Input: part model. Units: mm. Frame: model coordinates. Face numbers are marked on the shaded views. A direction names the side the tool comes from. Round coordinates to 2 decimals unless told otherwise and drop trailing zeros. Loops run counter-clockwise (first coordinate to the right, second up) from the corner with the lowest first, then second, coordinate; pieces in that order, holes last.
1) First-contact query: pin 1 (5 mm diameter, centred on y = -2, z = 13.5, fed in from -X); pin 2 (3 mm diameter, centred on y = -6.5, z = -5.5, fed in from -X); pin 3 (5 mm diameter, centred on y = -5, z = 2, fed in from +X). Flat tips, straight axial feed; report the tip coordinate or a pass-through.
2) Ray query, line 1 along X through (y, z) = (-1.5, 8.5); line 2 along Z through (x, y) = (-3.5, -2.5); line 3 along Z through (x, y) = (15.5, -7.25). Return the intervals inside material, ascending.
3) Access query for the marked faces 1, 2 and 3. Directions: +Z, -Z, +X, -X, +Y, -Y. A direction counts if a zero-diameter tool reaches every point of the face in a straight line with its end or side. Return the directions, or none.
4) Section C-C, the plane z = 2. Return loops of the section in (x, y).
5) Section B-B, the plane x = 16. Return loops of the section in (y, z).
6) Section A-A, the plane y = -7.5. Return loops of the section in (x, z).
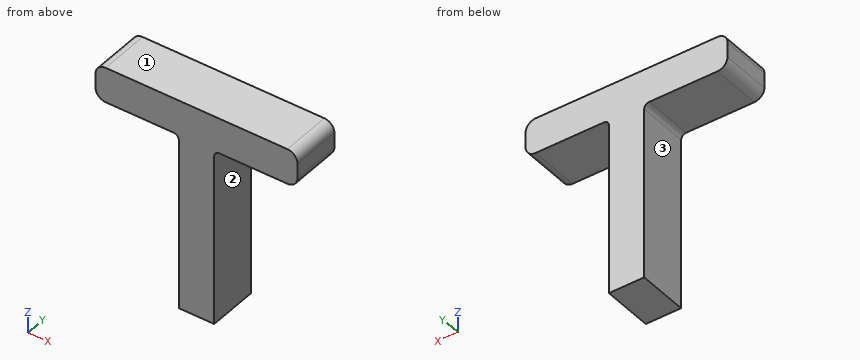
from build123d import *

# Parameters (mm, degrees)
F1_DEPTH = 10
F2_R     = 2
F3_R     = 1


with BuildPart() as f1:
    # F0 (on Front) → F1 (new body)
    with BuildSketch(Plane.XZ):
        Polygon((0, 16.178953), (0, -18.821047), (7, -18.821047), (7, 16.135083), (23.5, 16.135083), (23.5, 23.135083), (-16.5, 23.135083), (-16.5, 16.178953), (-5, 16.178953), align=None)
    extrude(amount=F1_DEPTH)

    # F2
    f2_edges = [f1.edges().sort_by_distance(p)[0] for p in [
        (-16.5, -5, 23.135083),
        (23.5, -5, 23.135083),
        (-16.5, -5, 16.178953),
        (23.5, -5, 16.135083),
    ]]
    fillet(f2_edges, radius=F2_R)

    # F3
    f3_edges = [f1.edges().sort_by_distance(p)[0] for p in [
        (0, -5, 16.178953),
        (7, -5, 16.135083),
    ]]
    fillet(f3_edges, radius=F3_R)


solid = f1.part
Final values:
1. pin 1: stops at x = -0.43
1. pin 2: stops at x = 0
1. pin 3: stops at x = 7
2. line 1: x = 0 to 7
2. line 2: z = 16.18 to 23.14
2. line 3: z = 16.14 to 23.14
3. face 1: +Z, +X, -X, +Y, -Y
3. face 2: -Z, +X, +Y, -Y
3. face 3: -Z, -X, +Y, -Y
4. outline: (0, -10) - (7, -10) - (7, 0) - (0, 0) - close
5. outline: (-10, 16.14) - (0, 16.14) - (0, 23.14) - (-10, 23.14) - close
6. outline: (-16.5, 18.18) arc R2 ccw to (-14.5, 16.18) - (-1, 16.18) arc R1 cw to (0, 15.18) - (0, -18.82) - (7, -18.82) - (7, 15.14) arc R1 cw to (8, 16.14) - (21.5, 16.14) arc R2 ccw to (23.5, 18.14) - (23.5, 21.14) arc R2 ccw to (21.5, 23.14) - (-14.5, 23.14) arc R2 ccw to (-16.5, 21.14) - close
